Source: CAD feature listing. Evaluate the final solid. Frame: model axes, mm. Coordinates: 2 decimals unless noted, no trailing zeros. Write each loop counter-clockwise with the first axis right and the second up, starting at its lowest first coordinate (ties: lowest second). Pieces come first, ordered by that corner, then holes. Notation, with made-up numbers: M 3.25,87.25 L 33.25,87.25 A18 cw 33.25,117.25 Z; hole C 24.5,35 d2. An arc over 180 degrees is marked long. Answer as CSV lines item,"result". Start each with the question number.
1. Contact query for a flat-ended pin moving along its axis: pin 1 Ø6 at (x, y) = (-43, 61) entering from +Z. Output: stop coordinate, or through.
2. Section A-A on x = -68. Return the cut outline in (y, z).
3. Line query: probe 1 along Y at (x, z) = (-38, 1.3); probe 2 along X at (y, z) = (66, 0.7); probe 3 along X at (y, z) = (37, 1.4). Output: solid intervals per line, ascending. Write a range as [from, to].
```python
from build123d import *

# Parameters (mm, degrees)
BOSS_EXTRUDE1_DEPTH = 2.54
CUT_EXTRUDE3_REACH  = 139.395
CUT_EXTRUDE4_DEPTH  = 77.978


with BuildPart() as part:
    # Sketch1 → Boss-Extrude1 (new body)
    with BuildSketch(Plane.XY):
        with BuildLine():
            Line((0, 0), (-114.3, 0))
            Line((-114.3, 0), (-114.3, 2.54))
            add(Edge.make_bspline(
                [(-114.3, 2.54), (-80.840252574, 11.511154975), (-76.2, 76.2)],
                knots=[0.188439876, 0.188439876, 0.188439876, 1.620106138, 1.620106138, 1.620106138], degree=2, weights=[1, 0.754546764, 1]))
            Line((-76.2, 76.2), (-50.8, 76.2))
            add(Edge.make_bspline(
                [(-50.8, 76.2), (-44.726222493, 11.346977385), (0, 2.54)],
                knots=[4.596431231, 4.596431231, 4.596431231, 6.031007642, 6.031007642, 6.031007642], degree=2, weights=[1, 0.753591079, 1]))
            Line((0, 2.54), (0, 0))
        make_face()
    extrude(amount=BOSS_EXTRUDE1_DEPTH)

    # Sketch4 → Cut-Extrude3 (cut, up to next)
    with BuildSketch(Plane.ZY.offset(114.3), mode=Mode.PRIVATE) as cut_extrude3_sk1:
        Polygon((2.54, 0), (0, 1.466469684), (0, 0), align=None)
    cut_extrude3_tool1 = extrude(cut_extrude3_sk1.sketch, amount=-CUT_EXTRUDE3_REACH, mode=Mode.PRIVATE) & part.part
    add(cut_extrude3_tool1.solids().sort_by_distance((-114.3, 0.488823, 0.846667))[0], mode=Mode.SUBTRACT)

    # Sketch5 → Cut-Extrude4 (cut)
    with BuildSketch(Plane.ZY.offset(114.3)):
        Polygon((0, 76.2), (2.54, 74.733530316), (2.54, 76.2), align=None)
    extrude(amount=-CUT_EXTRUDE4_DEPTH, mode=Mode.SUBTRACT)


solid = part.part
```
Values:
1,pin 1,"through"
2,outline,"M 0,2.54 L 1.47,0 L 76.2,0 L 74.73,2.54 Z"
3,probe 1,"[0.72, 34.23]"
3,probe 2,"[-77.29, -49.36]"
3,probe 3,"[-84.73, -39.49]"
